The figure shows three views and two pictorial views of one solid part (mm, origin at its lowest corner). Answer the questions. Give positions to 0.01 mm unless a question says otherwise; leave off trailing zeros. Loops run counter-clockwise (first coordinate to the right, second up) from the corner with the lowest first, then second, coordinate; pieces in that order, holes last.
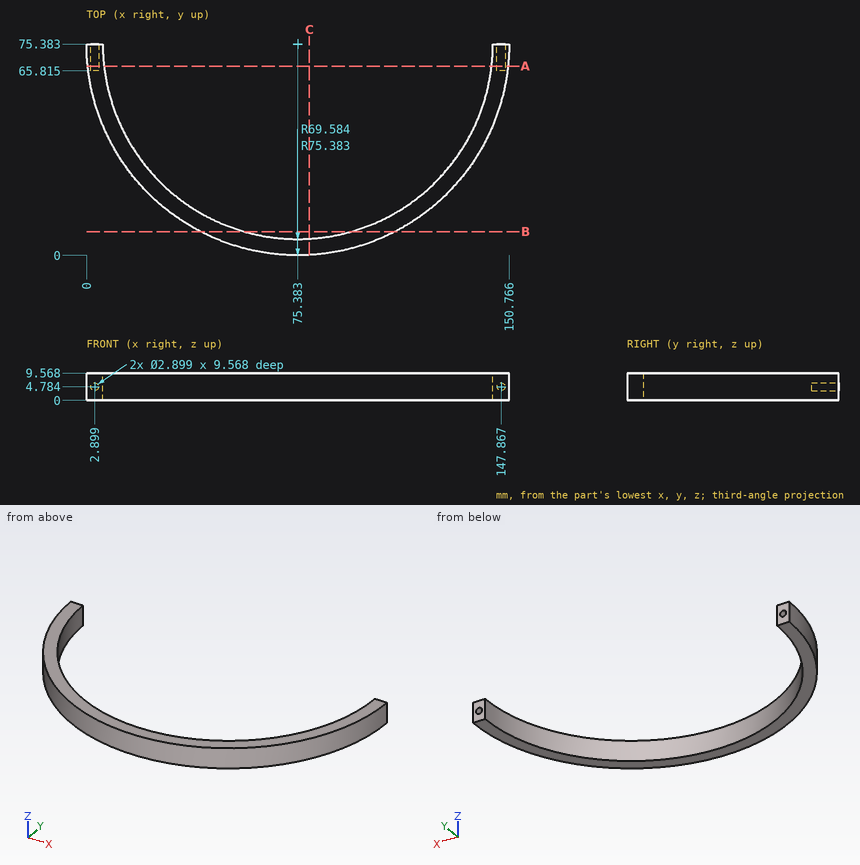
Q1. Section C-C on x = 79.5 is taken. Give the vertices of the cut face in (y, z).
Q2. Given pin 1 (1 mm diameter, centred on x = 73.5, z = 2, fed in from +Y); pin 2 (2.5 mm diameter, centred on x = 2.9, z = 4.78, fed in from +Y) (1 decimal); pin 3 (1 mm diameter, centred on y = 66, z = 8, fed in from +X), each flat-ended and moving along its own axis, determine where each tip first touches the part or whether it passes through.
Q3. Consider line 1 along X through (y, z) = (52.5, 7); line 2 along Y through (x, z) = (77, 5.5); line 3 along X through (y, z) = (30, 9) (1 decimal). Determine where each line is inside the solid, lowest interval first.
Q4. Section A-A on y = 67.5 is taken. Give the vertices of the cut face in (x, z).
Q5. Section B-B on y = 8.5 is taken. Give the vertices of the cut face in (x, z).
Check result:
1. outline: (0.11, 0) - (5.92, 0) - (5.92, 9.57) - (0.11, 9.57) - close
2. pin 1: stops at y = 5.84
2. pin 2: stops at y = 65.8
2. pin 3: stops at x = 150.24
3. line 1: x = 3.56 to 9.67, 141.1 to 147.21
3. line 2: y = 0.02 to 5.82
3. line 3: x = 15.2 to 22.6, 128.1 to 135.6
4. outline: (0.41, 0) - (6.25, 0) - (6.25, 9.57) - (0.41, 9.57) - close; (144.52, 0) - (150.35, 0) - (150.35, 9.57) - (144.52, 9.57) - close; hole circle Ø2.9 at (2.9, 4.78); hole circle Ø2.9 at (147.87, 4.78)
5. outline: (40.61, 0) - (56.18, 0) - (56.18, 9.57) - (40.61, 9.57) - close; (94.58, 0) - (110.16, 0) - (110.16, 9.57) - (94.58, 9.57) - close
